from build123d import *

# Parameters (mm, degrees)
ESQUISSE3_W                = 50
ESQUISSE3_H                = 60
BOSS_EXTRU_12_DEPTH        = 3
ESQUISSE4_R                = 17.25
ENL_V_MAT_EXTRU_1_DEPTH    = 5
ESQUISSE5_W                = 5
ESQUISSE5_H                = 10
ESQUISSE5_H_2              = 5
BOSS_EXTRU_13_DEPTH        = 3
R_P_TITION_LIN_AIRE1_COUNT = 5
R_P_TITION_LIN_AIRE1_PITCH = 10
ESQUISSE6_W                = 5
ESQUISSE6_H                = 5
BOSS_EXTRU_14_DEPTH        = 3
ESQUISSE7_W                = 2.5
ESQUISSE7_H                = 60
ENL_V_MAT_EXTRU_2_DEPTH    = 10


with BuildPart() as part:
    # Esquisse3 → Boss.-Extru.12 (new body)
    with BuildSketch(Plane.XY):
        with Locations((0, -10)):
            Rectangle(ESQUISSE3_W, ESQUISSE3_H)
    extrude(amount=BOSS_EXTRU_12_DEPTH)

    # Esquisse4 → Enlèv. mat.-Extru.1 (cut)
    with BuildSketch(Plane.XY.offset(3)):
        with Locations((0, -22)):
            Circle(ESQUISSE4_R)
    extrude(amount=-ENL_V_MAT_EXTRU_1_DEPTH, mode=Mode.SUBTRACT)

    # Esquisse5 → Boss.-Extru.13 (add)
    with BuildSketch(Plane.XY.offset(3)):
        with Locations((-20, 25)):
            Rectangle(ESQUISSE5_W, ESQUISSE5_H)
        with Locations((-20, -42.5)):
            Rectangle(ESQUISSE5_W, ESQUISSE5_H_2)
    boss_extru_13 = extrude(amount=-BOSS_EXTRU_13_DEPTH)

    # Répétition linéaire1: Boss.-Extru.13 ×5
    with Locations(*[(i * R_P_TITION_LIN_AIRE1_PITCH, 0, 0) for i in range(1, R_P_TITION_LIN_AIRE1_COUNT)]):
        add(boss_extru_13)

    # Esquisse6 → Boss.-Extru.14 (add)
    with BuildSketch(Plane.XY.offset(3)):
        with Locations((-5, -42.5)):
            Rectangle(ESQUISSE6_W, ESQUISSE6_H)
        with Locations((5, -42.5)):
            Rectangle(ESQUISSE6_W, ESQUISSE6_H)
    extrude(amount=-BOSS_EXTRU_14_DEPTH)

    # Esquisse7 → Enlèv. mat.-Extru.2 (cut)
    with BuildSketch(Plane.XY.offset(3)):
        with Locations((-23.75, -10)):
            Rectangle(ESQUISSE7_W, ESQUISSE7_H)
    extrude(amount=-ENL_V_MAT_EXTRU_2_DEPTH, mode=Mode.SUBTRACT)


solid = part.part
Model file for the job. Use its own axes, mm. A direction names the side the tool comes from. Give positions to 0.01 mm unless a question says otherwise; leave off trailing zeros. Order: outer loops, then holes, each group sorted by start corner. A loop starts at its lowest first (then second) coordinate and runs counter-clockwise, first axis right, second up. Notation, with made-up numbers: (-2, 76) - (14, 76) arc R10 cw to (14, 80) - close; hole circle Ø3 at (39.5, 38.5). An arc over 180 degrees is marked (long way). Return JSON: item names as keys, results as strings.
1) Cut at A-A, the plane y = 21.5. Give the cut face in (x, z).
Geometry says:
{"outline": "(-22.5, 0) - (-17.5, 0) - (-17.5, 3) - (-22.5, 3) - close; (-12.5, 0) - (-7.5, 0) - (-7.5, 3) - (-12.5, 3) - close; (-2.5, 0) - (2.5, 0) - (2.5, 3) - (-2.5, 3) - close; (7.5, 0) - (12.5, 0) - (12.5, 3) - (7.5, 3) - close; (17.5, 0) - (22.5, 0) - (22.5, 3) - (17.5, 3) - close"}
2) Pull direction X, two halves, no side cores. Call faces 1 (the flat face through (5, 20, 1)), 2 (the flat face through (22.5, 25, 2)), 3 (the flat face through (-22.5, -8, 2)): pulls with the +X half, pulls with the -X half, needs draft (parallel to the pull), parting line crosses it, or undercut.
Geometry says:
{"face 1": "undercut", "face 2": "pulls with the +X half", "face 3": "pulls with the -X half"}
3) 3-axis set-ups, long thin cutter, end or side, ignore diameter. For faces 4 (the flat face through (-7.5, 25, 2)), 5 (the flat face through (-15, -40, 1)), 6 (the flat face through (24, 20, 1)): which of +Z, -Z, +X, -X, +Y, -Y reach the whole face in a straight line?
Geometry says:
{"face 4": "+Z, -Z, +Y", "face 5": "+Z, -Z, -Y", "face 6": "+Z, -Z, +X, +Y"}
4) Cut at D-D, the plane y = -22. Give the cut face in (x, z).
Geometry says:
{"outline": "(-22.5, 0) - (-17.25, 0) - (-17.25, 3) - (-22.5, 3) - close; (17.25, 0) - (25, 0) - (25, 3) - (17.25, 3) - close"}
5) Cut at B-B, the plane x = 0. Give the cut face in (y, z), plus the area to 4 significant figures.
Geometry says:
{"outline": "(-45, 0) - (-39.25, 0) - (-39.25, 3) - (-45, 3) - close; (-4.75, 0) - (30, 0) - (30, 3) - (-4.75, 3) - close", "area": "121.5 mm²"}
6) Probe line 1 (X direction, y = 27, z = 1.6); line 2 (Y direction, x = 0, z = 1.4); line 3 (X direction, y = -29.5, z = 1.7). List the from-to ranges inside material, lowest first. Write a range as from..to.
Geometry says:
{"line 1": "-22.5..-17.5, -12.5..-7.5, -2.5..2.5, 7.5..12.5, 17.5..22.5", "line 2": "-45..-39.25, -4.75..30", "line 3": "-22.5..-15.53, 15.53..25"}
7) Flat gauge pins, fed straight in: P1, Ø1.5, axis at y = -42.5, z = 2, coming from the +X side; P2, Ø1.2, axis at x = 23.5, z = 1, coming from the +Y side. Where does each tip first touch, or does it go through?
Geometry says:
{"P1": "x = 22.5", "P2": "y = 20"}
